Drawing for the job (mm, zero at the part's lowest x, y, z). Give positions to 0.01 mm unless a question says otherwise; leave off trailing zeros. Write each loop counter-clockwise with the first axis right and the second up, starting at its lowest first coordinate (ties: lowest second). Pieces come first, ordered by that corner, then holes.
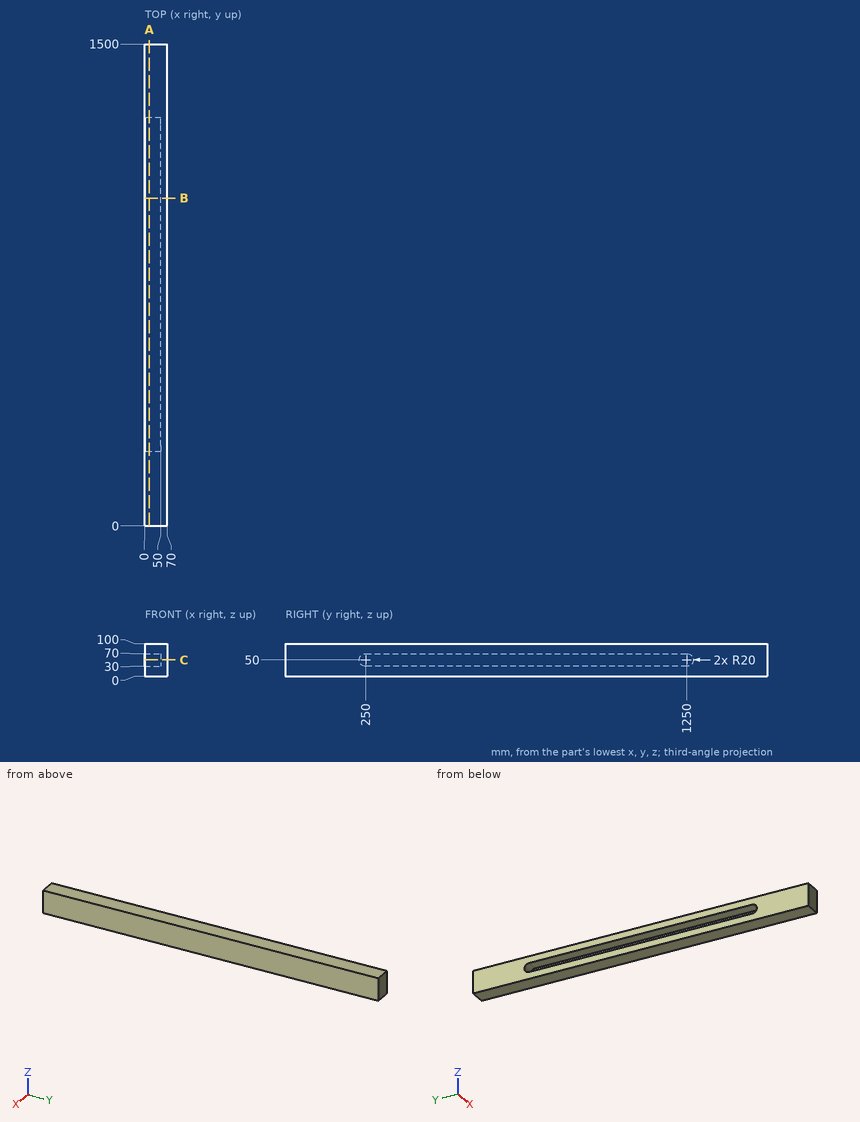
1. Slice it at B-B, the plane y = 1020. Write the cut outline in (x, z), and give its area (3 significant figures).
Calculated:
outline: (0, 0) - (70, 0) - (70, 100) - (0, 100) - (0, 70) - (50, 70) - (50, 30) - (0, 30) - close
area: 5,000 mm2
2. Probe probe 1 along Z at (x, y) = (43, 928.5); probe 2 along X at (y, z) = (1163, 64.5); probe 3 along Y at (x, z) = (26.5, 39). List the from-to ranges inside material, lowest first.
Calculated:
probe 1: z = 0 to 30, 70 to 100
probe 2: x = 50 to 70
probe 3: y = 0 to 233.3, 1266.7 to 1500
3. Slice it at A-A, the plane x = 14.5. Write the cut outline in (y, z), and give its area (3 significant figures).
Calculated:
outline: (0, 0) - (1500, 0) - (1500, 100) - (0, 100) - close; hole (250, 30) - (1250, 30) arc R20 ccw to (1250, 70) - (250, 70) arc R20 ccw to start
area: 109,000 mm2
4. Slice it at C-C, the plane z = 50. Write the cut outline in (x, y), and give its area (3 significant figures).
Calculated:
outline: (0, 0) - (70, 0) - (70, 1500) - (0, 1500) - (0, 1270) - (50, 1270) - (50, 230) - (0, 230) - close
area: 53,000 mm2
